Can you work these out from the model? Positions are in its coordinate system, mm. Face numbers are marked on the shaded views. A direction names the side the tool comes from. Give positions to 0.01 mm unless a question says otherwise; leave off trailing zeros. Order: outer loops, then holes, each group sorted by start corner. A loop starts at its lowest first (then second) coordinate and runs counter-clockwise, first axis right, second up. Notation, with made-up numbers: (18, 71) -> (30, 71) arc R18 cw to (30, 83) -> close; hole circle Ø3 at (-12, -20.5). An arc over 180 degrees is marked (long way). Answer as a JSON object with one key per item and string values.
Autodesk Inventor part; units mm, degrees
ref_plane "YZ Plane" through (0, 0, 0) normal (1, 0, 0) x (0, 1, 0)
ref_plane "XZ Plane" through (0, 0, 0) normal (0, 1, 0) x (-1, 0, 0)
ref_plane "XY Plane" through (0, 0, 0) normal (0, 0, 1) x (1, 0, 0)
sketch "Sketch1" plane through (0, 0, 0) normal (0, 1, 0) x (-1, 0, 0)
  circle A0 centre (0, 0) radius 34.95
  circle A1 centre (0, 0) radius 29.75
  line L0 (0, 0) -> (41.2193, -15.0026)
  line L1 (0, 0) -> (43.8647, 0) construction
  line L2 (0, 0) -> (47.0412, -17.1216)
  line L3 (0, 0) -> (50.0602, 0) construction
  line L4 (0, 0) -> (41.5964, 15.1399)
  line L5 (0, 0) -> (44.266, 0) construction
  point P0 (32.8423, 11.9536)
  point P1 (27.9559, 10.1751)
  point P2 (27.9559, -10.1751)
  point P3 (32.8423, -11.9536)
  dimension "d0" = 69.9
  dimension "d1" = 59.5
  dimension "d2" = 20
  dimension "d3" = 340
  dimension "d4" = 20
extrude "Extrusion1" add sketch "Sketch1" along normal blind 5 contours A0 L0 A1 L4 picked at (33.1379, 1.3525)
sketch "Sketch2" plane through (0, 0, 0) normal (1, 0, 0) x (0, 1, 0)
  line L0 (0, 0) -> (0, -1)
  line L1 (0, 10.1751) -> (0, -10.1751)
  line L2 (0, -1) -> (0, 1)
  line L3 (0, 0) -> (1, 0)
  line L4 (1, 0) -> (0, 1)
  line L5 (0, 0) -> (-1.5, 0)
  circle A0 centre (-1.5, 0) radius 3.25
  line L6 (1.75, 0) -> (2.25, 0)
  line L7 (2.25, 0) -> (1.3167, -1.6214)
  line L8 (2.25, 0) -> (1.3167, 1.6214)
  point P0 (0, 2.8831)
  point P1 (0, -2.8831)
  dimension "d7" = 1
  dimension "d8" = 2
  dimension "d9" = 1
  dimension "d16" = 1.5
  dimension "d17" = 6.5
  dimension "d18" = 0.5
sketch "Sketch3" plane through (0, 5, 0) normal (0, 1, 0) x (1, 0, 0)
  line L0 (0, 0) -> (-39.1232, 10.483)
  line L1 (0, 0) -> (40.5033, 0) construction
  line L2 (0, 0) -> (-4.9273, 0)
  arc A0 (-32.8423, 11.9536) -> (-32.8423, -11.9536) centre (0, 0) ccw
  line L3 (-33.7591, 9.0457) -> (-28.7363, 7.6999)
  arc A1 (-27.9559, 10.1751) -> (-27.9559, -10.1751) centre (0, 0) ccw
  circle A2 centre (-31.2477, 8.3728) radius 1.65
  circle A3 centre (-31.2477, -8.3728) radius 1.65
  dimension "d12" = 165
  dimension "d13" = 3.3
extrude "Extrusion3" cut sketch "Sketch3" against normal blind 100
extrude "Extrusion4" cut sketch "Sketch2" against normal blind 200 contours L3 L4 L1 A0 L0 | L1 L4 L3 | A0 L6 L7 | L8 L6 A0
properties part number "cable_jig_clamp"
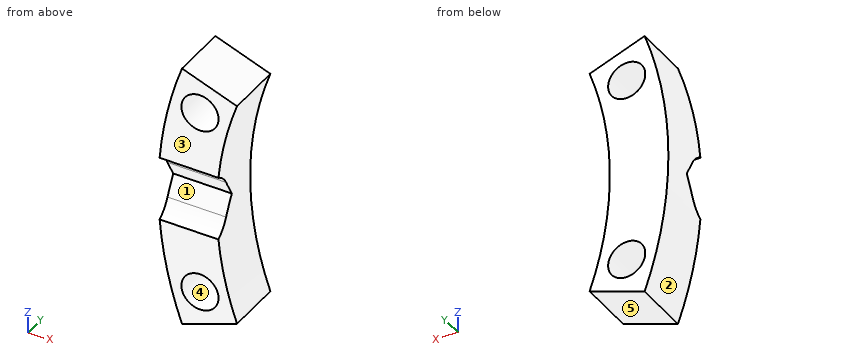
1. If we mould it in two halves opening along X, with no side actions, what happens to the marked faces 3, 4 and 5? For each: +X half, -X half, draft (parallel to the pull), parting line (faces both ways), or undercut.
Worked answers:
{"face 3": "draft", "face 4": "undercut", "face 5": "+X half"}
2. If we section it at D-D on z = -9.5: Please give me the cut outline in (x, y), then the cut area to 3 significant figures.
Worked answers:
{"outline": "(-33.63, 0) -> (-32.45, 0) -> (-32.45, 5) -> (-33.63, 5) -> close; (-30.04, 0) -> (-28.19, 0) -> (-28.19, 5) -> (-30.04, 5) -> close", "area": "15.2 mm²"}
3. If we section it at C-C on x = -29.25: Please give me the cut outline in (y, z), then the cut area to 3 significant figures.
Worked answers:
{"outline": "(0, -10.65) -> (5, -10.65) -> (5, -5.43) -> (0, -5.43) -> close; (0, 5.43) -> (5, 5.43) -> (5, 10.65) -> (0, 10.65) -> close", "area": "52.1 mm²"}
4. Please list where these lines run through material, in increasing order: L1, parallel to Z at x = -32.25, y = 2.9; L2, parallel to Z at x = -30, y = 2.15; L3, parallel to Z at x = -30.5, y = 1.5.
Worked answers:
{"L1": "-11.74 to -9.68, -7.06 to 7.06, 9.68 to 11.74", "L2": "-10.92 to -9.45, -7.29 to -0.17, 0.17 to 7.29, 9.45 to 10.92", "L3": "-11.1 to -9.84, -6.9 to -1.3, 1.3 to 6.9, 9.84 to 11.1"}
5. If we section it at A-A on x = -32.25: Please give me the cut outline in (y, z), then the cut area to 3 significant figures.
Worked answers:
{"outline": "(0, -11.74) -> (5, -11.74) -> (5, -9.68) -> (0, -9.68) -> close; (0, -7.06) -> (5, -7.06) -> (5, 7.06) -> (0, 7.06) -> (0, 2.88) arc R3.25 cw to (1.32, 1.62) -> (2.25, 0) -> (1.32, -1.62) arc R3.25 cw to (0, -2.88) -> close; (0, 9.68) -> (5, 9.68) -> (5, 11.74) -> (0, 11.74) -> close", "area": "83.4 mm²"}
6. For the marked faces 1 and 2, which set-ups out of +Z, -Z, +X, -X, +Y, -Y let a thin tool reach every point of the face, with its end or its side?
Worked answers:
{"face 1": "+X, -X, -Y", "face 2": "-X, +Y, -Y"}
7. If we section it at B-B on y = 1.9: Please give me the cut outline in (x, z), then the cut area to 3 significant figures.
Worked answers:
{"outline": "(-34.94, -0.61) arc R34.95 ccw to (-32.84, -11.95) -> (-27.96, -10.18) arc R29.75 cw to (-29.74, -0.61) -> close; (-34.94, 0.61) -> (-29.74, 0.61) arc R29.75 cw to (-27.96, 10.18) -> (-32.84, 11.95) arc R34.95 ccw to start; hole circle Ø3.3 at (-31.25, -8.37); hole circle Ø3.3 at (-31.25, 8.37)", "area": "94.0 mm²"}
8. Will these pins go through, and if not, where does the flat tip stop? pin 1 Ø3 at (y, z) = (2, -3) entering from -X; pin 2 Ø2 at (x, y) = (-31.5, 4.5) entering from +Z; pin 3 Ø2 at (y, z) = (4.5, -7.5) entering from +X.
Worked answers:
{"pin 1": "x = -34.92", "pin 2": "z = 11.83", "pin 3": "x = -28.51"}
